Here's how the part is built. I have some questions about the finished solid (model axes, mm). A direction names the side the tool comes from. Coordinates: 2 decimals unless noted, no trailing zeros. Loops run counter-clockwise (first coordinate to the right, second up) from the corner with the lowest first, then second, coordinate; pieces in that order, holes last. Notation, with made-up numbers: (79, -1.75) -> (129, -1.75) arc R24 ccw to (129, 26.25) -> close; hole circle Ø5 at (31.25, 43.25). An arc over 180 degrees is marked (long way). Answer as a JSON object with one key per item and string values. Group by question number.
1) I want a section at D-D (x = 20). Write out the boundary of the cut face in (y, z).
2) Which directions (+Z, -Z, +X, -X, +Y, -Y) give clear straight access to the entire face, cutting with the end or side of a thin tool? Please do faces 5 (the flat face through (46, 95, 5)), 6 (the flat face through (94.5, 47, 2)), 7 (the cylindrical face through (93.297, 1.141, 2.465)), 8 (the cylindrical face through (93.359, 93.297, 2.465)).
3) I want a section at A-A (y = -12.75). Write out the boundary of the cut face in (x, z), then the cut area to 3 significant figures.
4) If we mould it in two halves opening along Y, with no side actions, what happens to faces 1 (the flat face through (46, 117.25, 7)), 2 (the cylindrical face through (1.141, 1.203, 2.465)), 3 (the flat face through (0, 48, 2)), 4 (the cylindrical face through (92.766, -14.271, 7.465))? For each: +Y half, -Y half, draft (parallel to the pull), parting line (faces both ways), or undercut.
5) I need wall thicknesses on probe 1 along Y at (x, z) = (-0.25, 6.2); probe 2 along X at (y, z) = (87.91, 4) (3 decimals); probe 3 along Y at (x, z) = (87.91, 8) (3 decimals). Which ranges of each line are inside material? Lowest first, please. Write a range as [from, to].
6) I want a section at C-C (z = 2). Write out the boundary of the cut face in (x, y) (3 decimals).
7) I'm going to push flat-ended pins straight in: pin 1 (1.5 mm diameter, centred on x = 38, y = 58, fed in from -Z); pin 2 (1.5 mm diameter, centred on x = 48, z = 4, fed in from -Y); pin 3 (2.5 mm diameter, centred on y = 57, z = 2, fed in from +X). Where does each tip first touch, or does it pass through?
8) I want a section at B-B (y = 61). Write out the boundary of the cut face in (x, z), then the cut area to 3 significant figures.
```python
from build123d import *

# Parameters (mm, degrees)
SKETCH1_R           = 1.025
BOSS_EXTRUDE1_DEPTH = 5
SKETCH2_W           = 115
SKETCH2_H           = 140
SKETCH2_R           = 2.5
BOSS_EXTRUDE2_DEPTH = 5
CUT_EXTRUDE1_START  = -10
SKETCH3_R           = 1.025
CUT_EXTRUDE1_DEPTH  = 5


with BuildPart() as part:
    # Sketch1 → Boss-Extrude1 (new body)
    with BuildSketch(Plane.XY):
        with BuildLine():
            Line((4, 0), (90.5, 0))
            ThreePointArc((90.5, 0), (93.328427125, 1.171572875), (94.5, 4))
            Line((94.5, 4), (94.5, 90.5))
            ThreePointArc((94.5, 90.5), (93.328427125, 93.328427125), (90.5, 94.5))
            Line((90.5, 94.5), (4, 94.5))
            ThreePointArc((4, 94.5), (1.171572875, 93.328427125), (0, 90.5))
            Line((0, 90.5), (0, 4))
            ThreePointArc((0, 4), (1.171572875, 1.171572875), (4, 0))
        make_face()
        with Locations((6.59, 87.91)):
            Circle(SKETCH1_R, mode=Mode.SUBTRACT)
        with Locations((87.91, 87.91)):
            Circle(SKETCH1_R, mode=Mode.SUBTRACT)
        with Locations((6.59, 6.59)):
            Circle(SKETCH1_R, mode=Mode.SUBTRACT)
        with Locations((87.91, 6.59)):
            Circle(SKETCH1_R, mode=Mode.SUBTRACT)
    extrude(amount=BOSS_EXTRUDE1_DEPTH)

    # Sketch2 → Boss-Extrude2 (add)
    with BuildSketch(Plane.XY.offset(5)):
        with Locations((47.25, 47.25)):
            Rectangle(SKETCH2_W, SKETCH2_H)
        with Locations((94.75, 107.25)):
            Circle(SKETCH2_R, mode=Mode.SUBTRACT)
        with Locations((94.75, -12.75)):
            Circle(SKETCH2_R, mode=Mode.SUBTRACT)
        with Locations((-0.25, 107.25)):
            Circle(SKETCH2_R, mode=Mode.SUBTRACT)
        with Locations((-0.25, -12.75)):
            Circle(SKETCH2_R, mode=Mode.SUBTRACT)
    extrude(amount=BOSS_EXTRUDE2_DEPTH)

    # Sketch3 → Cut-Extrude1 (cut)
    with BuildSketch(Plane(origin=(0, 0, 0), x_dir=(-1, 0, 0), z_dir=(0, 0, -1)).offset(CUT_EXTRUDE1_START)):
        with Locations((-87.91, 6.59)):
            Circle(SKETCH3_R)
        with Locations((-6.59, 6.59)):
            Circle(SKETCH3_R)
        with Locations((-6.59, 87.91)):
            Circle(SKETCH3_R)
        with Locations((-87.91, 87.91)):
            Circle(SKETCH3_R)
    extrude(amount=CUT_EXTRUDE1_DEPTH, mode=Mode.SUBTRACT)


solid = part.part
```
Determined:
{
 "1": {"outline": "(-22.75, 5) -> (0, 5) -> (0, 0) -> (94.5, 0) -> (94.5, 5) -> (117.25, 5) -> (117.25, 10) -> (-22.75, 10) -> close"},
 "2": {"face 5": "-Z", "face 6": "-Z, +X, +Y, -Y", "face 7": "-Z, +X, -Y", "face 8": "-Z, +X, +Y"},
 "3": {"outline": "(-10.25, 5) -> (-2.75, 5) -> (-2.75, 10) -> (-10.25, 10) -> close; (2.25, 5) -> (92.25, 5) -> (92.25, 10) -> (2.25, 10) -> close; (97.25, 5) -> (104.75, 5) -> (104.75, 10) -> (97.25, 10) -> close", "area": "525 mm^2"},
 "4": {"face 1": "+Y half", "face 2": "-Y half", "face 3": "draft", "face 4": "undercut"},
 "5": {"probe 1": "[-22.75, -15.25], [-10.25, 104.75], [109.75, 117.25]", "probe 2": "[0, 5.565], [7.615, 86.885], [88.935, 94.5]", "probe 3": "[-22.75, 5.565], [7.615, 86.885], [88.935, 117.25]"},
 "6": {"outline": "(0, 4) arc R4 ccw to (4, 0) -> (90.5, 0) arc R4 ccw to (94.5, 4) -> (94.5, 90.5) arc R4 ccw to (90.5, 94.5) -> (4, 94.5) arc R4 ccw to (0, 90.5) -> close; hole circle Ø2.05 at (6.59, 6.59); hole circle Ø2.05 at (6.59, 87.91); hole circle Ø2.05 at (87.91, 6.59); hole circle Ø2.05 at (87.91, 87.91)"},
 "7": {"pin 1": "z = 0", "pin 2": "y = 0", "pin 3": "x = 94.5"},
 "8": {"outline": "(-10.25, 5) -> (0, 5) -> (0, 0) -> (94.5, 0) -> (94.5, 5) -> (104.75, 5) -> (104.75, 10) -> (-10.25, 10) -> close", "area": "1,050 mm^2"}
}
